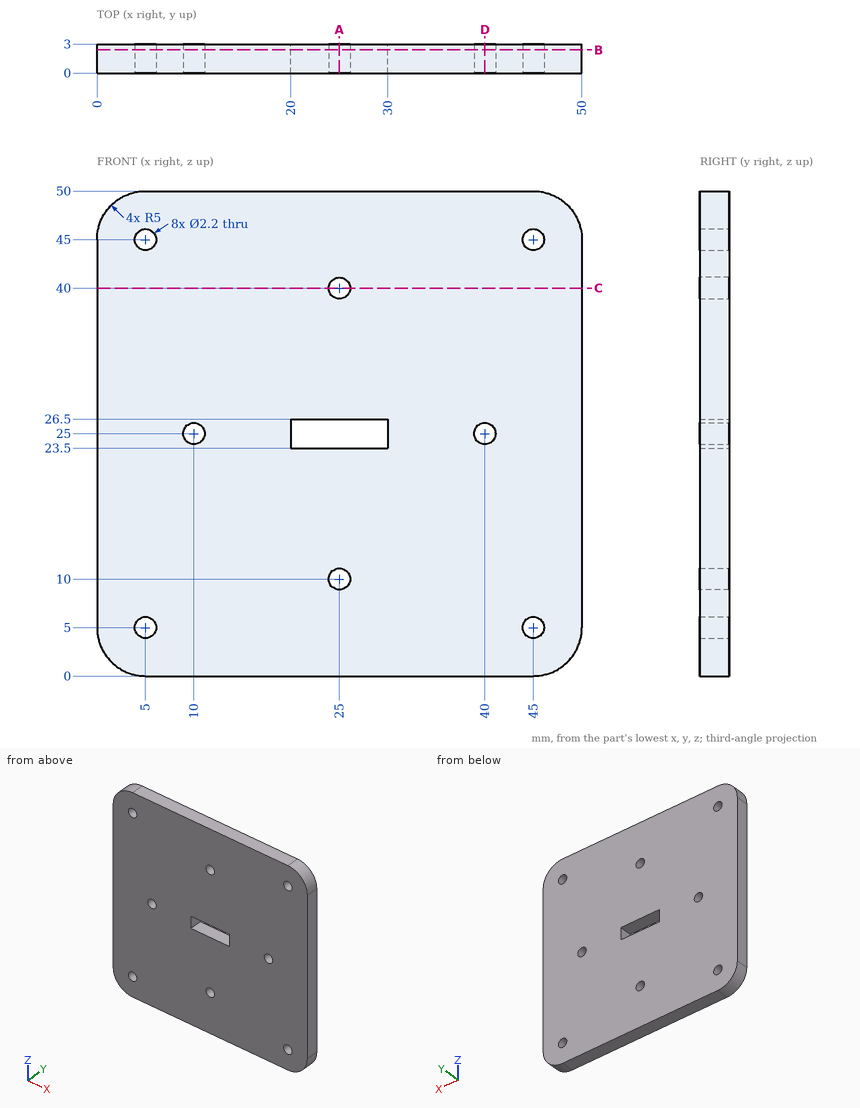
The figure shows three views and two pictorial views of one solid part (mm, origin at its lowest corner). Answer the questions. Coordinates: 2 decimals unless noted, no trailing zeros. Loops run counter-clockwise (first coordinate to the right, second up) from the corner with the lowest first, then second, coordinate; pieces in that order, holes last. Notation, with made-up numbers: (20.25, 29.25) -> (73.25, 29.25) arc R23 cw to (73.25, 40.25) -> close; hole circle Ø2 at (52, 10.25). An arc over 180 degrees is marked (long way). Return JSON: item names as keys, results as strings. Group by question number.
(1) A cutting plane is placed at C-C on z = 40. Write down the section's boundary in (x, y).
(2) A cutting plane is placed at B-B on y = 2.4. Count the separate pieces of the cut face and the enclosed holes in it, and give its area (3 significant figures).
(3) A cutting plane is placed at A-A on x = 25. Write down the section's boundary in (y, z), and give its area (3 significant figures).
(4) Find the intervals of material crossed by probe 1 along X at (y, z) = (1.5, 5); probe 2 along X at (y, z) = (2.2, 25); probe 3 along Z at (x, y) = (21, 1.2), in increasing order. Write a range as from..to.
(5) A cutting plane is placed at D-D on x = 40. Write down the section's boundary in (y, z).
(6) Given pin 1 Ø1.8 at (x, z) = (45, 5) entering from -Y, flat-ended and moving along its own axis, determine where the tip first touches the part or whether it passes through.
The answers:
{
 "1": {"outline": "(0, 0) -> (23.9, 0) -> (23.9, 3) -> (0, 3) -> close; (26.1, 0) -> (50, 0) -> (50, 3) -> (26.1, 3) -> close"},
 "2": {"separate pieces": "1", "enclosed holes": "9", "area": "2,420 mm^2"},
 "3": {"outline": "(0, 0) -> (3, 0) -> (3, 8.9) -> (0, 8.9) -> close; (0, 11.1) -> (3, 11.1) -> (3, 23.5) -> (0, 23.5) -> close; (0, 26.5) -> (3, 26.5) -> (3, 38.9) -> (0, 38.9) -> close; (0, 41.1) -> (3, 41.1) -> (3, 50) -> (0, 50) -> close", "area": "128 mm^2"},
 "4": {"probe 1": "x = 0..3.9, 6.1..43.9, 46.1..50", "probe 2": "x = 0..8.9, 11.1..20, 30..38.9, 41.1..50", "probe 3": "z = 0..23.5, 26.5..50"},
 "5": {"outline": "(0, 0) -> (3, 0) -> (3, 23.9) -> (0, 23.9) -> close; (0, 26.1) -> (3, 26.1) -> (3, 50) -> (0, 50) -> close"},
 "6": {"pin 1": "passes through"}
}
